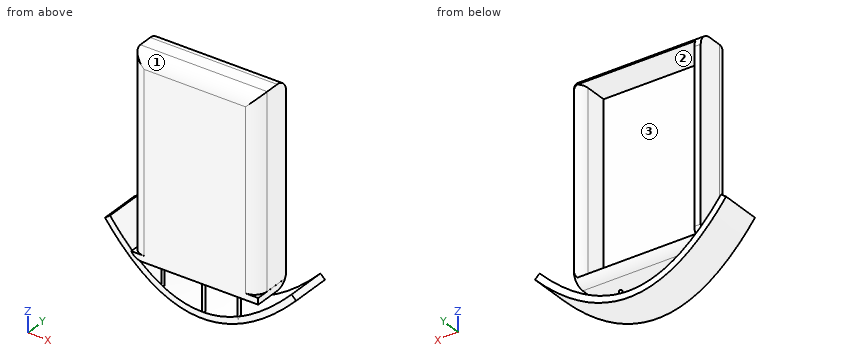
from build123d import *

# Parameters (mm, degrees)
BOSS_EXTRUDE1_DEPTH = 31
SKETCH5_W           = 90
SKETCH5_H           = 144.999999519
CUT_EXTRUDE2_DEPTH  = 26
SKETCH10_R          = 1.05
SKETCH10_R_2        = 1
BOSS_EXTRUDE3_DEPTH = 21
EXTRUDE_THIN2_START = -32
EXTRUDE_THIN2_DEPTH = 32
FILLET2_R           = 10
FILLET4_R           = 10
FILLET5_R           = 10
FILLET6_R           = 10
SKETCH15_R          = 1
BOSS_EXTRUDE4_DEPTH = 28


# Read off the part's stored shape, not the designer's step: Extrude-Thin2
with BuildPart() as part:
    # Sketch4 → Boss-Extrude1 (new body)
    with BuildSketch(Plane(origin=(0, 0, 0), x_dir=(1, 0, 0), z_dir=(0, 1, 0))):
        Polygon((-24.543123589, 51.393890829), (-24.485724986, 51.393890829), (-24.485724986, -98.606109173), (75.514275014, -98.606109173), (75.514275014, 51.393890827), (75.547211032, 51.393890827), (75.547211032, 56.393890829), (-24.543123589, 56.393890829), align=None)
    extrude(amount=BOSS_EXTRUDE1_DEPTH)

    # Sketch5 → Cut-Extrude2 (cut)
    with BuildSketch(Plane(origin=(0, 31, 0), x_dir=(1, 0, 0), z_dir=(0, 1, 0))):
        with Locations((25.514275014, -21.106109414)):
            Rectangle(SKETCH5_W, SKETCH5_H)
    extrude(amount=-CUT_EXTRUDE2_DEPTH, mode=Mode.SUBTRACT)

    # Sketch10 → Boss-Extrude3 (add)
    with BuildSketch(Plane(origin=(0, 0, -56.393890829), x_dir=(-1, 0, 0), z_dir=(0, 0, -1))):
        with Locations(Location((-55.547211032, 7, 0), (0, 0, 180))):
            Circle(SKETCH10_R)
        with Locations(Location((4.543123589, 7, 0), (0, 0, 180))):
            Circle(SKETCH10_R_2)
    extrude(amount=BOSS_EXTRUDE3_DEPTH)

    # Fillet2
    # the kernel refuses this fillet: 10 mm, written as the material it takes off along each edge
    with BuildSketch(Plane(origin=(-49.485724986, 31, 98.606109173), x_dir=(0, 0, -1), z_dir=(1, 0, 0))) as fillet2_piece_1:
        with BuildLine():
            CenterArc((FILLET2_R, -FILLET2_R), FILLET2_R, 90, 90)
            Line((0, -FILLET2_R), (0, 0))
            Line((0, 0), (FILLET2_R, 0))
        make_face()
    extrude(amount=150, mode=Mode.SUBTRACT)
    with BuildSketch(Plane(origin=(-24.485724986, 0, -51.393890829), x_dir=(0, 1, 0), z_dir=(0, 0, 1))) as fillet2_piece_2:
        with BuildLine():
            CenterArc((FILLET2_R, -FILLET2_R), FILLET2_R, 90, 90)
            Line((0, -FILLET2_R), (0, 0))
            Line((0, 0), (FILLET2_R, 0))
        make_face()
    extrude(amount=175.000000002, mode=Mode.SUBTRACT)
    with BuildSketch(Plane(origin=(-49.485724986, 0, 98.606109173), x_dir=(0, 0, -1), z_dir=(1, 0, 0))) as fillet2_piece_3:
        with BuildLine():
            CenterArc((FILLET2_R, FILLET2_R), FILLET2_R, 180, 90)
            Line((0, FILLET2_R), (0, 0))
            Line((0, 0), (FILLET2_R, 0))
        make_face()
    extrude(amount=150, mode=Mode.SUBTRACT)
    with BuildSketch(Plane(origin=(75.514275014, 0, 123.606109173), x_dir=(-1, 0, 0), z_dir=(0, 0, -1))) as fillet2_piece_4:
        with BuildLine():
            CenterArc((FILLET2_R, FILLET2_R), FILLET2_R, 180, 90)
            Line((0, FILLET2_R), (0, 0))
            Line((0, 0), (FILLET2_R, 0))
        make_face()
    extrude(amount=175, mode=Mode.SUBTRACT)

    # Fillet4
    # the kernel refuses this fillet: 10 mm, written as the material it takes off along each edge
    with BuildSketch(Plane(origin=(70.514275014, 31, -73.044525441), x_dir=(0, -1, 0), z_dir=(0, 0, 1))) as fillet4_piece_1_section:
        with BuildLine():
            CenterArc((8.660254038, 10), FILLET4_R, 210, 60)
            Line((0, 5), (0, 0))
            Line((0, 0), (8.660254038, 0))
        make_face()
    fillet4_piece_1 = extrude(amount=183.301269709, mode=Mode.PRIVATE)
    fillet4_piece_1 = split(fillet4_piece_1, bisect_by=Plane(origin=(71.836700468, 27.349745962, -51.393890827), z_dir=(0, 0, 1)), keep=Keep.TOP, mode=Mode.PRIVATE)
    fillet4_piece_1 = split(fillet4_piece_1, bisect_by=Plane(origin=(71.836700468, 27.349745962, 93.606109173), z_dir=(0, 0, -1)), keep=Keep.TOP, mode=Mode.PRIVATE)
    add(fillet4_piece_1, mode=Mode.SUBTRACT)

    # Fillet5
    # the kernel refuses this fillet: 10 mm, written as the material it takes off along each edge
    with BuildSketch(Plane(origin=(100.547211032, 31, -56.393890829), x_dir=(0, -1, 0), z_dir=(-1, 0, 0))) as fillet5_piece_1:
        with BuildLine():
            CenterArc((FILLET5_R, FILLET5_R), FILLET5_R, 180, 90)
            Line((0, FILLET5_R), (0, 0))
            Line((0, 0), (FILLET5_R, 0))
        make_face()
    extrude(amount=150.090334621, mode=Mode.SUBTRACT)

    # Fillet6
    # the kernel refuses this fillet: 10 mm, written as the material it takes off along each edge
    with BuildSketch(Plane(origin=(-24.543123589, -21.650635095, -56.393890829), x_dir=(0, 0, 1), z_dir=(0, 1, 0))) as fillet6_piece_1:
        with BuildLine():
            CenterArc((10, 8.660254038), FILLET6_R, 180, 60)
            Line((0, 8.660254038), (-0.2, 8.660254038))
            Line((-0.2, 8.660254038), (-0.2, 0))
            Line((-0.2, 0), (0, -0.2))
            ThreePointArc((0, -0.2), (2.5, -0.2), (4.9, -0.173205081))
            Line((4.9, -0.173205081), (5, 0))
        make_face()
    extrude(amount=64.301270189, mode=Mode.SUBTRACT)



with BuildPart() as body_2:
    # Extrude-Thin2 outline → Extrude-Thin2 (new body)
    with BuildSketch(Plane(origin=(0, 6.00667288, 0), x_dir=(-1, 0, 0), z_dir=(0, -1, 0)).offset(EXTRUDE_THIN2_START)):
        with BuildLine():
            Line((-101.106259616, 47.455416484), (-97.517183312, 43.974248393))
            add(Edge.make_bspline(
                [(-97.517183312, 43.974248393), (-90.947109033, 50.747979881), (-84.461523265, 56.594117718), (-71.690746068, 66.443323609), (-65.406461275, 70.445777381), (-53.067617331, 76.648178617), (-47.015104027, 78.848903051), (-35.121450693, 81.523458331), (-29.279693001, 82.000658953), (-17.700514878, 81.275147368), (-11.958520381, 80.072104414), (-0.470729692, 75.931508258), (5.275181576, 72.990557795), (16.783088845, 65.291546287), (22.542970532, 60.533005936), (34.041987864, 49.160363108), (39.780319498, 42.546980543), (45.491234369, 35.002570947)],
                knots=[0, 0, 0, 0, 0.125, 0.125, 0.25, 0.25, 0.375, 0.375, 0.5, 0.5, 0.625, 0.625, 0.75, 0.75, 0.875, 0.875, 1, 1, 1, 1], degree=3))
            Line((45.491234369, 35.002570947), (49.477851308, 38.020332599))
            add(Edge.make_bspline(
                [(-101.106259616, 47.455416484), (-20.540664315, 130.518360158), (49.477851308, 38.020332599)],
                knots=[0, 0, 0, 1, 1, 1], degree=2))
        make_face()
    extrude(amount=EXTRUDE_THIN2_DEPTH)


with BuildPart() as part_1:
    add(part.part)

    add(body_2.part)  # Boss-Extrude4 merges body 2
    # Sketch15 → Boss-Extrude4 (add)
    with BuildSketch(Plane(origin=(0, 0, -56.393890829), x_dir=(-1, 0, 0), z_dir=(0, 0, -1))):
        with Locations(Location((-27.678413699, 7, 0), (0, 0, 180))):
            Circle(SKETCH15_R)
    extrude(amount=BOSS_EXTRUDE4_DEPTH)


solid = part_1.part
Source: CAD feature listing. Evaluate the final solid. Frame: model axes, mm. Face numbers are marked on the shaded views. Round coordinates to 2 decimals unless told otherwise and drop trailing zeros. Loops run counter-clockwise (first coordinate to the right, second up) from the corner with the lowest first, then second, coordinate; pieces in that order, holes last. Notation, with made-up numbers: (57.5, 76) - (106.5, 76) arc R24 ccw to (106.5, 110) - close; hole circle Ø1 at (62.25, 51.5). An arc over 180 degrees is marked (long way). Write item = value, one per line. Start each with the question number.
Item 1: Section query B-B on z = -61.5. Count the separate pieces of the cut face and the enclosed holes in it, plus the area to 3 significant figures.
Item 2: Mould query, pull axis X, two halves, no side actions, for the marked faces 1, 2 and 3. Classes: released by +X, released by -X, zero draft, split by the parting line, or undercut.
Item 3: Material intervals for line 1 (X direction, y = 11, z = 2.5); line 2 (Z direction, x = 50, y = 21); line 3 (Z direction, x = 3.5, y = 27.5), sorted ascending.
Item 4: Section query A-A on z = 12. Output: boundary loops of the cut face in (x, y), plus the area to 3 significant figures.
Item 5: First-contact query: pin 1 Ø1 at (x, y) = (62.5, 25.5) entering from +Z; pin 2 Ø3 at (x, z) = (9.5, 53) entering from +Y; pin 3 Ø4 at (y, z) = (31.5, 79) entering from -X. Flat tips, straight axial feed; report the tip coordinate or a pass-through.
Results list:
q1.separate_pieces = 5
q1.enclosed_holes = 0
q1.area = 505 mm²
q2.face_1 = zero draft
q2.face_2 = undercut
q2.face_3 = undercut
q3.line_1 = -24.49 to -19.49, 70.51 to 75.51
q3.line_2 = -82.85 to -77.55, -56.39 to -51.39, 93.61 to 98.61
q3.line_3 = -82.33 to -76.96, -53.99 to -51.39, 93.61 to 96.21
q4.outline = (-24.49, 10) arc R10 ccw to (-14.49, 0) - (65.51, 0) arc R10 ccw to (75.51, 10) - (75.51, 31) arc R10 ccw to (70.51, 22.34) - (70.51, 5) - (-19.49, 5) - (-19.49, 31) - (-24.49, 31) - close
q4.area = 704 mm²
q5.pin_1 = 97.77
q5.pin_2 = 5
q5.pin_3 = -24.49
